```python
from build123d import *

# Parameters (mm, degrees)
EXTRUDE_1_DEPTH = 0.5


with BuildPart() as part:
    # 草图1 → 凸台-拉伸1 (new, symmetric)
    with BuildSketch(Plane.XY):
        with BuildLine():
            ThreePointArc((-0.975265745, 11.076672173), (-4.475265745, 7.576672173), (-0.975265745, 4.076672173))
            ThreePointArc((-0.975265745, 4.076672173), (0.524734255, 2.576672173), (-0.975265745, 1.076672173))
            ThreePointArc((-0.975265745, 1.076672173), (-7.475265745, 7.576672173), (-0.975265745, 14.076672173))
            ThreePointArc((-0.975265745, 14.076672173), (0.524734255, 12.576672173), (-0.975265745, 11.076672173))
        make_face()
        with BuildLine():
            ThreePointArc((-0.975265745, 11.576672173), (-4.975265745, 7.576672173), (-0.975265745, 3.576672173))
            ThreePointArc((-0.975265745, 3.576672173), (0.024734255, 2.576672173), (-0.975265745, 1.576672173))
            ThreePointArc((-0.975265745, 1.576672173), (-6.975265745, 7.576672173), (-0.975265745, 13.576672173))
            ThreePointArc((-0.975265745, 13.576672173), (0.024734255, 12.576672173), (-0.975265745, 11.576672173))
        make_face(mode=Mode.SUBTRACT)
    extrude(amount=EXTRUDE_1_DEPTH, both=True)


solid = part.part
```
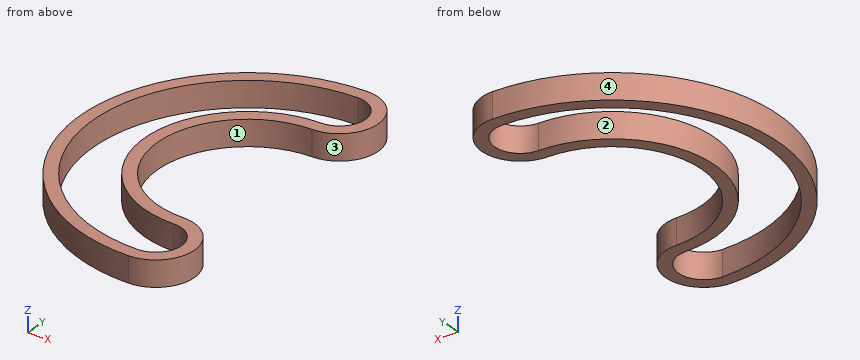
Could you check a few things on this model? Use its own coordinates, in mm. Face numbers are marked on the shaded views. A direction names the side the tool comes from. Coordinates: 2 decimals unless noted, no trailing zeros. Loops run counter-clockwise (first coordinate to the right, second up) from the corner with the lowest first, then second, coordinate; pieces in that order, holes last.
1) Which directions (+Z, -Z, +X, -X, +Y, -Y) give clear straight access to the entire face, cutting with the end or side of a thin tool? Please do the marked faces 1 and 2.
Reported:
face 1: +Z, -Z, +X
face 2: +Z, -Z
2) Please list where these lines run through material, in increasing order: line 1 along Y through (x, z) = (-4, 0.25); line 2 along Y through (x, z) = (-0.5, 0.2); line 3 along X through (y, z) = (12, 0.2).
Reported:
line 1: y = 1.82 to 2.39, 4.96 to 5.82, 9.34 to 10.19, 12.76 to 13.33
line 2: y = 1.15 to 1.7, 3.46 to 4, 11.15 to 11.7, 13.46 to 14
line 3: x = -5.74 to -5.03, -0.16 to 0.41
3) Thinking about a two-plate mould opening in Y: for the marked faces 3 and 4, which applies, released by +Y, released by -Y, zero draft, split by the parting line, or undercut?
Reported:
face 3: undercut
face 4: split by the parting line
4) Imagine slicing it at C-C (x = -5.75). List the corners of the cut face in (y, z) for me.
Reported:
outline: (3.17, -0.5) - (3.94, -0.5) - (3.94, 0.5) - (3.17, 0.5) - close; (11.21, -0.5) - (11.99, -0.5) - (11.99, 0.5) - (11.21, 0.5) - close
5) Imagine slicing it at B-B (y = 5.75). List the corners of the cut face in (x, z) for me.
Reported:
outline: (-7.21, -0.5) - (-6.69, -0.5) - (-6.69, 0.5) - (-7.21, 0.5) - close; (-4.53, -0.5) - (-3.96, -0.5) - (-3.96, 0.5) - (-4.53, 0.5) - close
6) Imagine slicing it at D-D (x = -4.25). List the corners of the cut face in (y, z) for me.
Reported:
outline: (1.96, -0.5) - (2.55, -0.5) - (2.55, 0.5) - (1.96, 0.5) - close; (5.28, -0.5) - (6.34, -0.5) - (6.34, 0.5) - (5.28, 0.5) - close; (8.81, -0.5) - (9.87, -0.5) - (9.87, 0.5) - (8.81, 0.5) - close; (12.6, -0.5) - (13.19, -0.5) - (13.19, 0.5) - (12.6, 0.5) - close
7) Imagine slicing it at A-A (z = 0). List the corners of the cut face in (x, y) for me.
Reported:
outline: (-0.98, 1.08) arc R1.5 ccw to (-0.98, 4.08) arc R3.5 cw to (-0.98, 11.08) arc R1.5 ccw to (-0.98, 14.08) arc R6.5 ccw to start; hole (-0.98, 1.58) arc R1 ccw to (-0.98, 3.58) arc R4 cw to (-0.98, 11.58) arc R1 ccw to (-0.98, 13.58) arc R6 ccw to start
